The listing builds one solid part. Answer for the finished solid, in the listing's coordinates (mm). Give positions to 0.01 mm unless a question says otherwise; leave off trailing zeros. Write each loop counter-clockwise with the first axis right and the second up, starting at its lowest first coordinate (ties: lowest second). Pieces come first, ordered by that corner, then holes. Notation, with made-up numbers: (-22, 22) - (-9, 22) arc R17 ccw to (-9, 29) - close; hole circle Ø1 at (9.5, 68). An arc over 180 degrees is marked (long way). Return JSON: item names as keys, results as strings.
from build123d import *

# Parameters (mm, degrees)
F7_COUNT = 25
F7_ANGLE = 345.6


with BuildPart() as f1:
    # F0 (on Front) → F1 (revolve)
    with BuildSketch(Plane.XZ):
        Polygon((5.5470483679, 18.0012998082), (0.0122273423, 12.4664593884), (-0.0058063755, 4.0821318731), (-5.763291413, 4.0821318731), (-5.763291413, 0), (0, 0), (16.8451661991, 0), (16.8451661991, 4.0821318731), (11.0818887877, 4.0821318731), (11.0818887877, 12.4664787826), align=None)
    revolve(axis=Axis((8.4225830996, 0, 0), (-1, 0, 0)))


with BuildPart() as f6:
    # F5 (on face) → F6 section 0
    with BuildSketch(Plane(origin=(-5.5200079815, 0, 5.5199886393), x_dir=(0, -1, 0), z_dir=(-0.70710802, 0, 0.7071055423)), mode=Mode.PRIVATE) as f6_s0:
        Polygon((0, 16.6512121101), (0, 12.7288497215), (1.3675010996, 12.7288497215), (2.4401100818, 16.6512121101), align=None)
    loft([f6_s0.sketch, Vertex(23.5484112532, 0, 0)])


with BuildPart() as f7_1:
    # F7: instance of F6
    add(f6.part.rotate(Axis((16.8451661991, 0, 0), (-1, 0, 0)), 1 * F7_ANGLE / (F7_COUNT - 1)))


with BuildPart() as f7_2:
    # F7: instance of F6
    add(f6.part.rotate(Axis((16.8451661991, 0, 0), (-1, 0, 0)), 2 * F7_ANGLE / (F7_COUNT - 1)))


with BuildPart() as f7_3:
    # F7: instance of F6
    add(f6.part.rotate(Axis((16.8451661991, 0, 0), (-1, 0, 0)), 3 * F7_ANGLE / (F7_COUNT - 1)))


with BuildPart() as f7_4:
    # F7: instance of F6
    add(f6.part.rotate(Axis((16.8451661991, 0, 0), (-1, 0, 0)), 4 * F7_ANGLE / (F7_COUNT - 1)))


with BuildPart() as f7_5:
    # F7: instance of F6
    add(f6.part.rotate(Axis((16.8451661991, 0, 0), (-1, 0, 0)), 5 * F7_ANGLE / (F7_COUNT - 1)))


with BuildPart() as f7_6:
    # F7: instance of F6
    add(f6.part.rotate(Axis((16.8451661991, 0, 0), (-1, 0, 0)), 6 * F7_ANGLE / (F7_COUNT - 1)))


with BuildPart() as f7_7:
    # F7: instance of F6
    add(f6.part.rotate(Axis((16.8451661991, 0, 0), (-1, 0, 0)), 7 * F7_ANGLE / (F7_COUNT - 1)))


with BuildPart() as f7_8:
    # F7: instance of F6
    add(f6.part.rotate(Axis((16.8451661991, 0, 0), (-1, 0, 0)), 8 * F7_ANGLE / (F7_COUNT - 1)))


with BuildPart() as f7_9:
    # F7: instance of F6
    add(f6.part.rotate(Axis((16.8451661991, 0, 0), (-1, 0, 0)), 9 * F7_ANGLE / (F7_COUNT - 1)))


with BuildPart() as f7_10:
    # F7: instance of F6
    add(f6.part.rotate(Axis((16.8451661991, 0, 0), (-1, 0, 0)), 10 * F7_ANGLE / (F7_COUNT - 1)))


with BuildPart() as f7_11:
    # F7: instance of F6
    add(f6.part.rotate(Axis((16.8451661991, 0, 0), (-1, 0, 0)), 11 * F7_ANGLE / (F7_COUNT - 1)))


with BuildPart() as f7_12:
    # F7: instance of F6
    add(f6.part.rotate(Axis((16.8451661991, 0, 0), (-1, 0, 0)), 12 * F7_ANGLE / (F7_COUNT - 1)))


with BuildPart() as f7_13:
    # F7: instance of F6
    add(f6.part.rotate(Axis((16.8451661991, 0, 0), (-1, 0, 0)), 13 * F7_ANGLE / (F7_COUNT - 1)))


with BuildPart() as f7_14:
    # F7: instance of F6
    add(f6.part.rotate(Axis((16.8451661991, 0, 0), (-1, 0, 0)), 14 * F7_ANGLE / (F7_COUNT - 1)))


with BuildPart() as f7_15:
    # F7: instance of F6
    add(f6.part.rotate(Axis((16.8451661991, 0, 0), (-1, 0, 0)), 15 * F7_ANGLE / (F7_COUNT - 1)))


with BuildPart() as f7_16:
    # F7: instance of F6
    add(f6.part.rotate(Axis((16.8451661991, 0, 0), (-1, 0, 0)), 16 * F7_ANGLE / (F7_COUNT - 1)))


with BuildPart() as f7_17:
    # F7: instance of F6
    add(f6.part.rotate(Axis((16.8451661991, 0, 0), (-1, 0, 0)), 17 * F7_ANGLE / (F7_COUNT - 1)))


with BuildPart() as f7_18:
    # F7: instance of F6
    add(f6.part.rotate(Axis((16.8451661991, 0, 0), (-1, 0, 0)), 18 * F7_ANGLE / (F7_COUNT - 1)))


with BuildPart() as f7_19:
    # F7: instance of F6
    add(f6.part.rotate(Axis((16.8451661991, 0, 0), (-1, 0, 0)), 19 * F7_ANGLE / (F7_COUNT - 1)))


with BuildPart() as f7_20:
    # F7: instance of F6
    add(f6.part.rotate(Axis((16.8451661991, 0, 0), (-1, 0, 0)), 20 * F7_ANGLE / (F7_COUNT - 1)))


with BuildPart() as f7_21:
    # F7: instance of F6
    add(f6.part.rotate(Axis((16.8451661991, 0, 0), (-1, 0, 0)), 21 * F7_ANGLE / (F7_COUNT - 1)))


with BuildPart() as f7_22:
    # F7: instance of F6
    add(f6.part.rotate(Axis((16.8451661991, 0, 0), (-1, 0, 0)), 22 * F7_ANGLE / (F7_COUNT - 1)))


with BuildPart() as f7_23:
    # F7: instance of F6
    add(f6.part.rotate(Axis((16.8451661991, 0, 0), (-1, 0, 0)), 23 * F7_ANGLE / (F7_COUNT - 1)))


with BuildPart() as f7_24:
    # F7: instance of F6
    add(f6.part.rotate(Axis((16.8451661991, 0, 0), (-1, 0, 0)), 24 * F7_ANGLE / (F7_COUNT - 1)))


with BuildPart() as f1_1:
    add(f1.part)

    # F8: cut F6, F7_1, F7_2, F7_3, F7_4, F7_5, F7_6, F7_7, F7_8, F7_9, F7_10, F7_11, F7_12, F7_13, F7_14, F7_15, F7_16, F7_17, F7_18, F7_19, F7_20, F7_21, F7_22, F7_23, F7_24
    add(f6.part, mode=Mode.SUBTRACT)
    add(f7_1.part, mode=Mode.SUBTRACT)
    add(f7_2.part, mode=Mode.SUBTRACT)
    add(f7_3.part, mode=Mode.SUBTRACT)
    add(f7_4.part, mode=Mode.SUBTRACT)
    add(f7_5.part, mode=Mode.SUBTRACT)
    add(f7_6.part, mode=Mode.SUBTRACT)
    add(f7_7.part, mode=Mode.SUBTRACT)
    add(f7_8.part, mode=Mode.SUBTRACT)
    add(f7_9.part, mode=Mode.SUBTRACT)
    add(f7_10.part, mode=Mode.SUBTRACT)
    add(f7_11.part, mode=Mode.SUBTRACT)
    add(f7_12.part, mode=Mode.SUBTRACT)
    add(f7_13.part, mode=Mode.SUBTRACT)
    add(f7_14.part, mode=Mode.SUBTRACT)
    add(f7_15.part, mode=Mode.SUBTRACT)
    add(f7_16.part, mode=Mode.SUBTRACT)
    add(f7_17.part, mode=Mode.SUBTRACT)
    add(f7_18.part, mode=Mode.SUBTRACT)
    add(f7_19.part, mode=Mode.SUBTRACT)
    add(f7_20.part, mode=Mode.SUBTRACT)
    add(f7_21.part, mode=Mode.SUBTRACT)
    add(f7_22.part, mode=Mode.SUBTRACT)
    add(f7_23.part, mode=Mode.SUBTRACT)
    add(f7_24.part, mode=Mode.SUBTRACT)


solid = f1_1.part
Item 1: Consider L1, parallel to Z at x = 5, y = 3; L2, parallel to Z at x = 6.5, y = 9; L3, parallel to Z at x = 9.25, y = -11. Determine where each line is inside the solid, lowest interval first.
Answer below:
{"L1": "z = -17.19 to -15.79, -13.32 to 13.09, 15.79 to 17.19", "L2": "z = -14.48 to -12.39, -9.96 to 9.58, 12.38 to 14.48", "L3": "z = -9.1 to -7.01, -5.18 to -3.38, -2.1 to -0.44, 0.69 to 2.32, 3.57 to 5.27, 6.98 to 8.88"}
Item 2: Flat-ended cylindrical pins translate along their axes: P1, Ø12, axis at y = -13, z = 12.5, coming from the -X side; P2, Ø5, axis at y = -11.5, z = -12.5, coming from the -X side; P3, Ø5, axis at x = 13, z = 11, coming from the +Y side; P4, Ø1, axis at x = -1, y = 8, coming from the -Z side. Find the tip coordinate at first contact, or state that the pin passes through.
Answer below:
{"P1": "stops at x = 0.01", "P2": "stops at x = 2.03", "P3": "stops at y = 7.51", "P4": "passes through"}
Item 3: A cutting plane is placed at A-A on x = -1.5. Determine the outline of the cut face in (y, z).
Answer below:
{"outline": "circle Ø8.16 at (0, 0)"}
